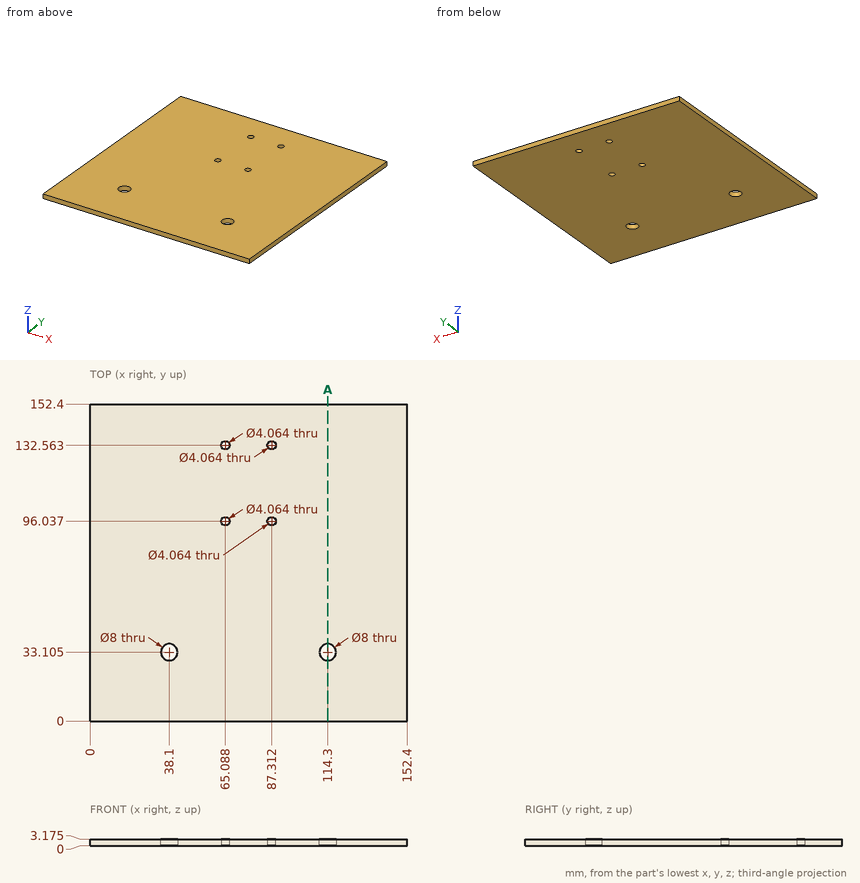
Geometry check sheet. Reference: drawing and pictorial views, mm from the part's lowest x, y, z. Round coordinates to 2 decimals unless told otherwise and drop trailing zeros. Loops run counter-clockwise (first coordinate to the right, second up) from the corner with the lowest first, then second, coordinate; pieces in that order, holes last. Notation, with made-up numbers: M 59.5,12 L 76.5,12 A34 cw 76.5,49 Z; hole C 22.5,22 d5. An arc over 180 degrees is marked long. One line per item, written item: value.
(1) Depth check by flat-ended pin: pin 1 Ø2.5 at (x, y) = (65.09, 96.04) entering from +Z. Enter the tip coordinate at first touch or a pass-through.
Computed values:
pin 1: passes through
(2) Sectioned sample at A-A, the plane x = 114.3. Record the cut outline in (y, z) (1 decimal).
Computed values:
outline: M 0,0 L 29.1,0 L 29.1,3.2 L 0,3.2 Z; M 37.1,0 L 152.4,0 L 152.4,3.2 L 37.1,3.2 Z
(3) Thickness scan on line 1 (Y direction, x = 38.1, z = 1.65) (1 decimal); line 2 (Y direction, x = 66, z = 3) (1 decimal); line 3 (Y direction, x = 112.5, z = 1.4) (1 decimal). Record the ranges inside material, lowest first.
Computed values:
line 1: y = 0 to 29.1, 37.1 to 152.4
line 2: y = 0 to 94.2, 97.9 to 130.7, 134.4 to 152.4
line 3: y = 0 to 29.5, 36.7 to 152.4
